Answer from the drawing. Dimensions are ordinates in mm from the lowest x, y and z of the part. A direction names the side the tool comes from. Give positions to 0.01 mm unless a question says otherwise; leave off trailing zeros. Order: outer loops, then holes, each group sorted by start corner. A loop starts at its lowest first (then second) coordinate and runs counter-clockwise, first axis right, second up. Notation, with made-up numbers: (17.25, 12.5) -> (47.25, 12.5) arc R16 ccw to (47.25, 32.5) -> close; hole circle Ø7 at (83.25, -12.75). An arc over 180 degrees is marked (long way). One line per question, with ' | ' between items. Start each with the question number.
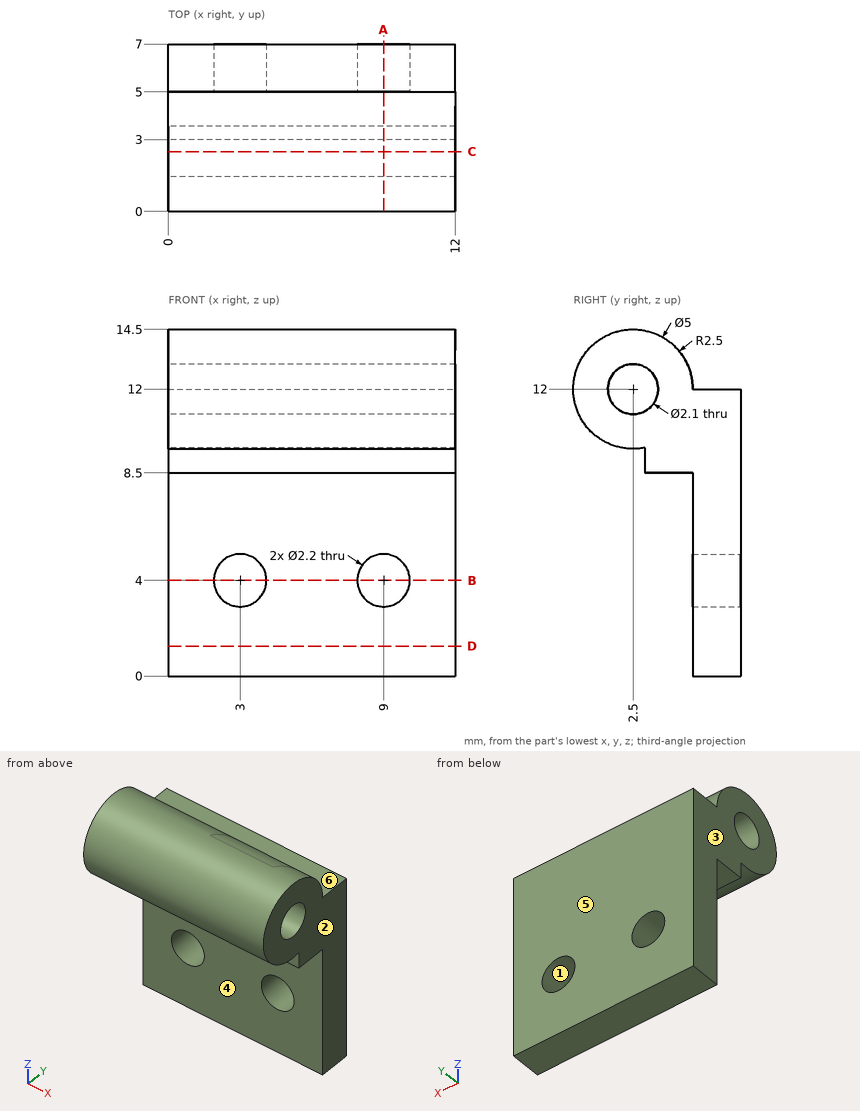
(1) The part is cut by section C-C on y = 2.5. Determine the outline of the cut face in (x, z), plus the area to 3 significant figures.
(2) The part is cut by section B-B on z = 4. Determine the outline of the cut face in (x, y).
(3) Determine the mould class of the marked faces 1, 2 and 3 for opening direction X: pulls with the +X half, pulls with the -X half, needs draft (parallel to the pull), parting line crosses it, or undercut.
(4) Consider line 1 (X direction, y = 6.4, z = 4); line 2 (X direction, y = 5.75, z = 3.5); line 3 (Y direction, x = 4, z = 5.5). Determine where each line is inside the solid, lowest interval first.
(5) The part is cut by section D-D on z = 1.25. Determine the outline of the cut face in (x, y), plus the area to 3 significant figures.
(6) Given P1, Ø1.6, axis at x = 5.5, y = 3.5, coming from the -Z side; P2, Ø4, axis at x = 9, z = 6, coming from the -Y side; P3, Ø3, axis at x = 6, y = 1, coming from the -Z side, each flat-ended and moving along its own axis, determine where each tip first touches the part or whether it passes through.
(7) For the marked faces 4, 5 and 6, determine the directions among +Z, -Z, +X, -X, +Y, -Y from which every point of the face is accessible in a straight line to the end or side of a thin tool.
(8) The part is cut by section A-A on x = 9. Determine the outline of the cut face in (y, z).
Result sheet:
1) outline: (0, 9.5) -> (12, 9.5) -> (12, 10.95) -> (0, 10.95) -> close; (0, 13.05) -> (12, 13.05) -> (12, 14.5) -> (0, 14.5) -> close | area: 34.8 mm^2
2) outline: (0, 5) -> (1.9, 5) -> (1.9, 7) -> (0, 7) -> close; (4.1, 5) -> (7.9, 5) -> (7.9, 7) -> (4.1, 7) -> close; (10.1, 5) -> (12, 5) -> (12, 7) -> (10.1, 7) -> close
3) face 1: undercut | face 2: pulls with the +X half | face 3: pulls with the -X half
4) line 1: x = 0 to 1.9, 4.1 to 7.9, 10.1 to 12 | line 2: x = 0 to 2.02, 3.98 to 8.02, 9.98 to 12 | line 3: y = 5 to 7
5) outline: (0, 5) -> (12, 5) -> (12, 7) -> (0, 7) -> close | area: 24.0 mm^2
6) P1: stops at z = 8.5 | P2: stops at y = 5 | P3: stops at z = 9.5
7) face 4: -Z, +X, -X, -Y | face 5: +Z, -Z, +X, -X, +Y | face 6: +Z, +X, -X, +Y
8) outline: (3, 8.5) -> (5, 8.5) -> (5, 5.1) -> (7, 5.1) -> (7, 12) -> (5, 12) arc R2.5 ccw (long way) to (3, 9.55) -> close; (5, 0) -> (7, 0) -> (7, 2.9) -> (5, 2.9) -> close; hole circle Ø2.1 at (2.5, 12)
